Verification items for this drawing (mm, ordinates from the low corner). Give positions to 0.01 mm unless a question says otherwise; leave off trailing zeros. Order: outer loops, then holes, each group sorted by start corner. A loop starts at its lowest first (then second) coordinate and runs counter-clockwise, first axis right, second up. Notation, with made-up numbers: M 6,44.5 L 12,44.5 A30 cw 12,74.5 Z; hole C 58.5,71 d2. An arc over 180 degrees is marked long. One line per question, with ' | ' between items. Start each with the question number.
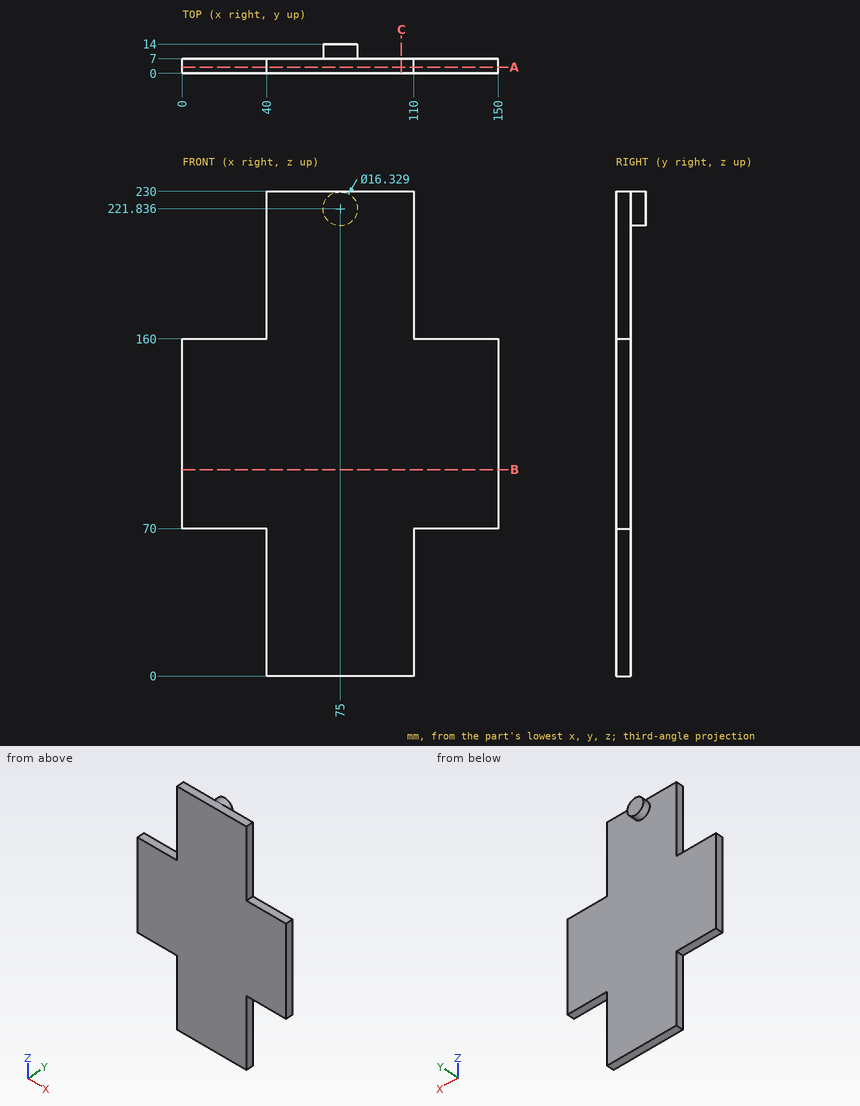
Item 1: Material ranges on line 1 along X through (y, z) = (0.5, 178); line 2 along Z through (x, y) = (9, 6.25); line 3 along Y through (x, z) = (47.5, 16), recorded low to high.
Item 2: Cross-section at C-C, the plane x = 104. Record the cut outline in (y, z), plus the area to 3 significant figures.
Item 3: Depth check by flat-ended pin: pin 1 (5.5 mm diameter, centred on x = 17, y = 2, fed in from +Z); pin 2 (6 mm diameter, centred on x = 119.5, y = 2, fed in from -Z); pin 3 (8 mm diameter, centred on y = 5.5, z = 199, fed in from -X); pin 4 (8 mm diameter, centred on x = 49, y = 12, fed in from -Z). Enter the tip coordinate at first touch or a pass-through.
Item 4: Cross-section at A-A, the plane y = 3. Record the cut outline in (x, z).
Item 5: Cross-section at B-B, the plane z = 98. Record the cut outline in (x, y), plus the area to 3 significant figures.
Outcome:
1) line 1: x = 40 to 110 | line 2: z = 70 to 160 | line 3: y = 0 to 7
2) outline: M 0,0 L 7,0 L 7,230 L 0,230 Z | area: 1,610 mm²
3) pin 1: stops at z = 160 | pin 2: stops at z = 70 | pin 3: stops at x = 40 | pin 4: passes through
4) outline: M 0,70 L 40,70 L 40,0 L 110,0 L 110,70 L 150,70 L 150,160 L 110,160 L 110,230 L 40,230 L 40,160 L 0,160 Z
5) outline: M 0,0 L 150,0 L 150,7 L 0,7 Z | area: 1,050 mm²
